Could you check a few things on this model? Use its own coordinates, in mm. Face numbers are marked on the shaded views. A direction names the side the tool comes from. Give positions to 0.01 mm unless a question says otherwise; leave off trailing zeros. Loops run counter-clockwise (first coordinate to the right, second up) from the corner with the lowest first, then second, coordinate; pieces in that order, holes last. Notation, with made-up numbers: (57, -24) -> (89, -24) arc R21 ccw to (89, -8) -> close; hole circle Ø2 at (-28, -18). An arc over 180 degrees is marked (long way). Write item = value, one per line. Start each with the question number.
1) I need wall thicknesses on probe 1 along X at (y, z) = (15.5, 41); probe 2 along Z at (x, y) = (54, 14); probe 3 along X at (y, z) = (2, -9.5). Which ranges of each line are inside material? Lowest first, please. Write a range as from..to.
2) I'm going to push flat-ended pins straight in: pin 1 Ø12.5 at (x, y) = (69.5, 15.5) entering from +Z; pin 2 Ø3 at (y, z) = (17.5, -9) entering from -X; pin 3 Ø9.5 at (y, z) = (27, -8) entering from +X. Where does each tip first touch, or does it pass through?
3) I want a section at A-A (y = 30). List the corners of the cut face in (x, z) for me, and give its area (3 significant figures).
4) I want a section at B-B (z = 2). List the corners of the cut face in (x, y) for me, and give its area (3 significant figures).
5) On a 3-axis mill with a long thin cutter (end or side, diameter ignored), from which of +Z, -Z, +X, -X, +Y, -Y can I reach the whole of each face in a straight line? I mean the marked faces 1, 2 and 3. Say none if no direction works.
6) I want a section at C-C (x = 66). List the corners of the cut face in (y, z) for me, and give its area (3 significant figures).
from build123d import *

# Parameters (mm, degrees)
F6_DEPTH = 47.244


# Not quite as in the source:
# - a feature of the source that left no trace in its solid (it failed there, or was rolled back) is left out


with BuildPart() as f6:
    # F0 (on Front) → F6 (new body)
    with BuildSketch(Plane.XZ):
        Polygon((52.8543624759, 44.45), (-29.6956375241, 44.45), (-29.6956375241, -6.35), (-23.3456375241, -6.35), (-23.3456375241, -12.7), (52.8543624759, -12.7), (52.8543624759, 6.35), (78.2543624759, 6.35), (78.2543624759, 12.7), (52.8543624759, 12.7), align=None)
    extrude(amount=-F6_DEPTH)


solid = f6.part
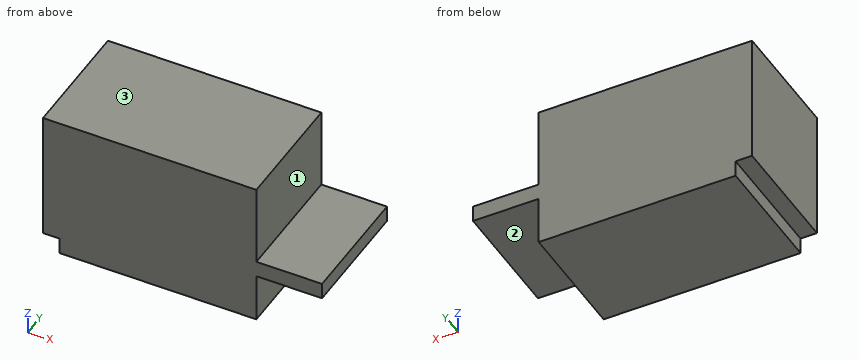
Answer list:
q1.probe_1 = -29.7..52.85
q1.probe_2 = 6.35..12.7
q1.probe_3 = -23.35..52.85
q2.pin_1 = 12.7
q2.pin_2 = -23.35
q2.pin_3 = 52.85
q3.outline = (-29.7, -6.35) -> (-23.35, -6.35) -> (-23.35, -12.7) -> (52.85, -12.7) -> (52.85, 6.35) -> (78.25, 6.35) -> (78.25, 12.7) -> (52.85, 12.7) -> (52.85, 44.45) -> (-29.7, 44.45) -> close
q3.area = 4,840 mm^2
q4.outline = (-29.7, 0) -> (52.85, 0) -> (52.85, 47.24) -> (-29.7, 47.24) -> close
q4.area = 3,900 mm^2
q5.face_1 = +Z, +X, +Y, -Y
q5.face_2 = -Z, +X, +Y, -Y
q5.face_3 = +Z, +X, -X, +Y, -Y
q6.outline = (0, 6.35) -> (47.24, 6.35) -> (47.24, 12.7) -> (0, 12.7) -> close
q6.area = 300 mm^2
